Part model, mm, in its own coordinate system. Face numbers are marked on the shaded views. A direction names the side the tool comes from. Round coordinates to 2 decimals unless told otherwise and drop trailing zeros. Loops run counter-clockwise (first coordinate to the right, second up) from the corner with the lowest first, then second, coordinate; pieces in that order, holes last. Notation, with made-up numbers: (32, -8.5) - (79, -8.5) arc R21 ccw to (79, 14.5) - close; hole circle Ø3 at (-21, 39). An arc over 180 degrees is marked (long way). Put each result on its own line as item: value.
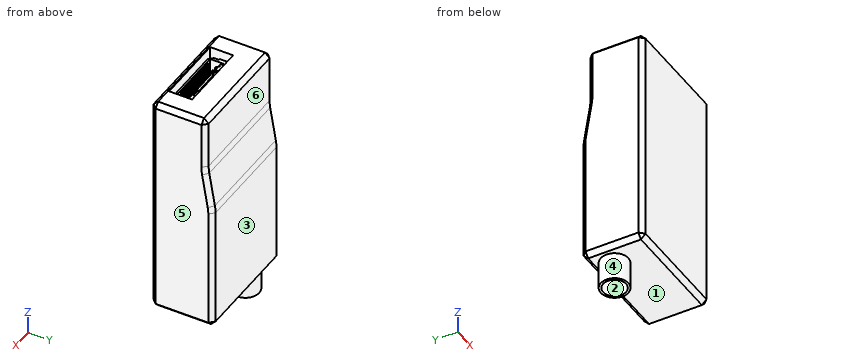
from build123d import *

# Parameters (mm, degrees)
BOSS_EXTRUDE1_DEPTH = 25
CHAMFER1_SIZE       = 1
SKETCH4_W           = 15.5
SKETCH4_H           = 5
CUT_EXTRUDE1_DEPTH  = 10
SKETCH5_W           = 1
SKETCH5_H           = 0.55
BOSS_EXTRUDE2_DEPTH = 8
CUT_EXTRUDE2_DEPTH  = 10
SKETCH7_W           = 0.3
SKETCH7_H           = 0.3
BOSS_EXTRUDE3_DEPTH = 10
SKETCH8_R           = 3
SKETCH8_R_2         = 2.5
BOSS_EXTRUDE4_DEPTH = 6


with BuildPart() as part:
    # Sketch3 → Boss-Extrude1 (new body)
    with BuildSketch(Plane(origin=(0, 0, 0), x_dir=(0, 0, -1), z_dir=(1, 0, 0))):
        with BuildLine():
            Line((0, 0), (-49, 0))
            Line((-49, 0), (-49, 12))
            Line((-49, 12), (-37.827625303, 12))
            ThreePointArc((-37.827625303, 12), (-37.002819988, 12.03407324), (-36.18363543, 12.136060762))
            Line((-36.18363543, 12.136060762), (-28.81636457, 13.363939238))
            ThreePointArc((-28.81636457, 13.363939238), (-27.997180012, 13.46592676), (-27.172374697, 13.5))
            Line((-27.172374697, 13.5), (0, 13.5))
            Line((0, 13.5), (0, 0))
        make_face()
    extrude(amount=BOSS_EXTRUDE1_DEPTH)

    # Chamfer1
    chamfer1_edges = [part.edges().sort_by_distance(p)[0] for p in [
        (0, 12.75, 32.5),
        (0, 13.46592676, 27.997180012),
        (0, 13.5, 13.586187349),
        (0, 6.75, 0),
        (25, 13.46592676, 27.997180012),
        (12.5, 0, 0),
        (12.5, 0, 49),
        (12.5, 12, 49),
        (12.5, 13.5, 0),
        (25, 12.75, 32.5),
        (25, 12.03407324, 37.002819988),
        (25, 12, 43.413812651),
        (25, 6, 49),
        (25, 0, 24.5),
        (25, 6.75, 0),
        (0, 0, 24.5),
        (25, 13.5, 13.586187349),
        (0, 6, 49),
        (0, 12, 43.413812651),
        (0, 12.03407324, 37.002819988),
    ]]
    chamfer(chamfer1_edges, length=CHAMFER1_SIZE)

    # Sketch4 → Cut-Extrude1 (cut)
    with BuildSketch(Plane.XY.offset(49)):
        with Locations((12.5, 3.731572294)):
            Rectangle(SKETCH4_W, SKETCH4_H)
    extrude(amount=-CUT_EXTRUDE1_DEPTH, mode=Mode.SUBTRACT)

    # Sketch5 → Boss-Extrude2 (add)
    with BuildSketch(Plane.XY.offset(39)):
        Polygon((20.186366737, 6.162059048), (4.813633263, 6.162059048), (4.813633263, 3.362059048), (5.1, 3.362059048), (5.1, 2.250733439), (5.988674392, 1.362059048), (19.011325608, 1.362059048), (19.9, 2.250733439), (19.9, 3.362059048), (20.186366737, 3.362059048), align=None)
        Polygon((8.1, 6.062059048), (16.9, 6.062059048), (16.9, 4.562059048), (15.516884386, 4.562059048), (15.030478648, 4.762059048), (9.969521352, 4.762059048), (9.483115614, 4.562059048), (8.1, 4.562059048), align=None, mode=Mode.SUBTRACT)
        with Locations((17.75, 5.405243542)):
            Rectangle(SKETCH5_W, SKETCH5_H, mode=Mode.SUBTRACT)
        with Locations((19.15, 5.399458355)):
            Rectangle(SKETCH5_W, SKETCH5_H, mode=Mode.SUBTRACT)
        with Locations((5.85, 5.399458355)):
            Rectangle(SKETCH5_W, SKETCH5_H, mode=Mode.SUBTRACT)
        with Locations((7.25, 5.405243542)):
            Rectangle(SKETCH5_W, SKETCH5_H, mode=Mode.SUBTRACT)
    extrude(amount=BOSS_EXTRUDE2_DEPTH)

    # Sketch6 → Cut-Extrude2 (cut)
    with BuildSketch(Plane.XY.offset(47)):
        Polygon((12.29, 4.267126877), (12.71, 4.267126877), (12.71, 3.897126877), (12.81, 3.897126877), (12.81, 4.267126877), (12.91, 4.267126877), (12.91, 3.897644042), (13.01, 3.897644042), (13.01, 4.267126877), (13.91, 4.267126877), (13.91, 3.897126877), (14.01, 3.897126877), (14.01, 4.267126877), (14.11, 4.267126877), (14.11, 3.897644042), (14.21, 3.897644042), (14.21, 4.267126877), (15.11, 4.267126877), (15.11, 3.897126877), (15.21, 3.897126877), (15.21, 4.267126877), (15.31, 4.267126877), (15.31, 3.897644042), (15.41, 3.897644042), (15.41, 4.267126877), (16.31, 4.267126877), (16.31, 3.897126877), (16.41, 3.897126877), (16.41, 4.267126877), (16.51, 4.267126877), (16.51, 3.897644042), (16.61, 3.897644042), (16.61, 4.267126877), (17.51, 4.267126877), (17.51, 3.897126877), (17.61, 3.897126877), (17.61, 4.267126877), (17.71, 4.267126877), (17.71, 3.897644042), (17.81, 3.897644042), (17.81, 4.267126877), (18.18, 4.267126877), (18.18, 4.477126877), (18.4, 4.477126877), (18.4, 4.267126877), (18.9, 4.267126877), (18.9, 4.767126877), (19.3, 4.767126877), (19.3, 1.767126877), (5.7, 1.767126877), (5.7, 4.767126877), (6.1, 4.767126877), (6.1, 4.267126877), (6.6, 4.267126877), (6.6, 4.477126877), (6.82, 4.477126877), (6.82, 4.267126877), (7.19, 4.267126877), (7.19, 3.897644042), (7.29, 3.897644042), (7.29, 4.267126877), (7.39, 4.267126877), (7.39, 3.897126877), (7.49, 3.897126877), (7.49, 4.267126877), (8.39, 4.267126877), (8.39, 3.897644042), (8.49, 3.897644042), (8.49, 4.267126877), (8.59, 4.267126877), (8.59, 3.897126877), (8.69, 3.897126877), (8.69, 4.267126877), (9.59, 4.267126877), (9.59, 3.897644042), (9.69, 3.897644042), (9.69, 4.267126877), (9.79, 4.267126877), (9.79, 3.897126877), (9.89, 3.897126877), (9.89, 4.267126877), (10.79, 4.267126877), (10.79, 3.897644042), (10.89, 3.897644042), (10.89, 4.267126877), (10.99, 4.267126877), (10.99, 3.897126877), (11.09, 3.897126877), (11.09, 4.267126877), (11.99, 4.267126877), (11.99, 3.897644042), (12.09, 3.897644042), (12.09, 4.267126877), (12.19, 4.267126877), (12.19, 3.897126877), (12.29, 3.897126877), align=None)
    extrude(amount=-CUT_EXTRUDE2_DEPTH, mode=Mode.SUBTRACT)

    # Sketch7 → Boss-Extrude3 (add)
    with BuildSketch(Plane.XY.offset(47)):
        with Locations((7.13, 1.917126877)):
            Rectangle(SKETCH7_W, SKETCH7_H)
        with Locations((8.31, 1.917126877)):
            Rectangle(SKETCH7_W, SKETCH7_H)
        with Locations((9.49, 1.917126877)):
            Rectangle(SKETCH7_W, SKETCH7_H)
        with Locations((10.67, 1.917126877)):
            Rectangle(SKETCH7_W, SKETCH7_H)
        with Locations((11.85, 1.917126877)):
            Rectangle(SKETCH7_W, SKETCH7_H)
        with Locations((13.03, 1.917126877)):
            Rectangle(SKETCH7_W, SKETCH7_H)
        with Locations((14.21, 1.917126877)):
            Rectangle(SKETCH7_W, SKETCH7_H)
        with Locations((15.39, 1.917126877)):
            Rectangle(SKETCH7_W, SKETCH7_H)
        with Locations((16.57, 1.917126877)):
            Rectangle(SKETCH7_W, SKETCH7_H)
    extrude(amount=-BOSS_EXTRUDE3_DEPTH)

    # Sketch8 → Boss-Extrude4 (add)
    with BuildSketch(Plane(origin=(0, 0, 0), x_dir=(-1, 0, 0), z_dir=(0, 0, -1))):
        with Locations((-4.714743405, 8.886764937)):
            Circle(SKETCH8_R)
        with Locations((-4.714743405, 8.886764937)):
            Circle(SKETCH8_R_2, mode=Mode.SUBTRACT)
    extrude(amount=BOSS_EXTRUDE4_DEPTH)


solid = part.part
1. Band-saw the part on C-C (y = 10.5). List the corners of the cut face in (x, z).
A:
outline: (0, 1) - (1, 0) - (2.19, 0) - (2.19, -6) - (2.8, -6) - (2.8, 0) - (6.62, 0) - (6.62, -6) - (7.24, -6) - (7.24, 0) - (24, 0) - (25, 1) - (25, 48) - (24, 49) - (1, 49) - (0, 48) - close
2. Band-saw the part on A-A (x = 22.5). List the corners of the cut face in (y, z), plus the area to 3 significant figures.
A:
outline: (0, 1) - (1, 0) - (12.5, 0) - (13.5, 1) - (13.5, 27.17) arc R10 ccw to (13.36, 28.82) - (12.14, 36.18) arc R10 cw to (12, 37.83) - (12, 48) - (11, 49) - (1, 49) - (0, 48) - close
area: 635 mm²
3. Band-saw the part on B-B (z = 33). List the corners of the cut face in (x, y), plus the area to 3 significant figures.
A:
outline: (0, 1) - (1, 0) - (24, 0) - (25, 1) - (25, 11.65) - (24, 12.67) - (1, 12.67) - (0, 11.65) - close
area: 315 mm²
4. Pin check, flat tips, straight feed: P1, Ø5, axis at x = 13, y = 6.5, coming from the -Z side; P2, Ø2.5, axis at x = 11, y = 4, coming from the +Z side. Stop position of each tip, or through.
A:
P1: stops at z = 0
P2: stops at z = 47
5. Two-plate mould, pull along Y, no slides. Class the marked faces 1, 2 and 3: pulls with the +Y half, pulls with the -Y half, needs draft (parallel to the pull), parting line crosses it, or undercut.
A:
face 1: needs draft
face 2: undercut
face 3: pulls with the +Y half
6. Band-saw the part on D-D (z = -1). List the corners of the cut face in (x, y).
A:
outline: circle Ø6 at (4.71, 8.89); hole circle Ø5 at (4.71, 8.89)
7. Tool access for the marked faces 4, 5 and 6: list every direction of +Z, -Z, +X, -X, +Y, -Y with a clear straight run to the whole face (end or side of a thin tool).
A:
face 4: -Z
face 5: +Z, -Z, +X, +Y, -Y
face 6: +Z, +X, -X, +Y
8. Probe line 1 along X through (y, z) = (9, -1); line 2 along Z through (x, y) = (21.5, 4.5); line 3 along Z through (x, y) = (10.5, 5). List the from-to ranges inside material, lowest first. Write a range as [from, to].
A:
line 1: x = [1.72, 2.22], [7.21, 7.71]
line 2: z = [0, 49]
line 3: z = [0, 39]
